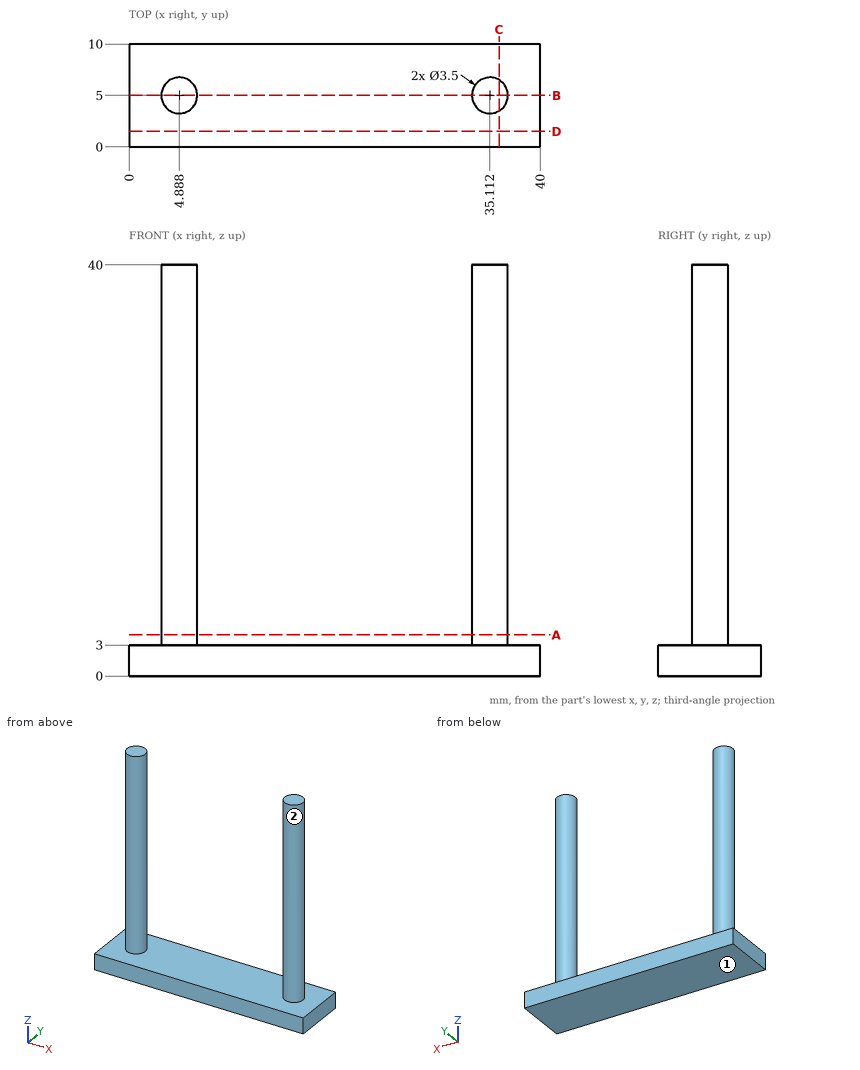
The drawing under review shows one solid part. Ordinate dimensions are in mm from its lowest x, y, z. Give positions to 0.01 mm unless a question says otherwise; leave off trailing zeros. Write each loop counter-clockwise with the first axis right and the second up, starting at its lowest first coordinate (ties: lowest second). Pieces come first, ordered by that corner, then holes.
1. Add section A-A, the plane z = 4. Write out the cut boundary in (x, y).
2. Add section C-C, the plane x = 36. Write out the cut boundary in (y, z).
3. Wall thickness on L1, parallel to Z at x = 15, y = 7.5; L2, parallel to Y at x = 35, z = 30; L3, parallel to X at y = 4.25, z = 23: over which ranges is each line inside the solid? List them lowest first.
4. For P1, Ø6, axis at y = 8.5, z = 35, coming from the +X side; P2, Ø12, axis at x = 17.5, z = 13, coming from the +Y side; P3, Ø5, axis at y = 7.5, z = 16.5, coming from the -X side, all flat-tipped, find the tip position at first contact; note any pin that passes through.
5. Draft analysis for pull direction X (two halves, no side actions). For the marked faces 1 and 2, state which applies: +X half, -X half, draft (parallel to the pull), parting line (faces both ways), or undercut.
6. Add section B-B, the plane y = 5. Write out the cut boundary in (x, z).
7. Add section D-D, the plane y = 1.5. Write out the cut boundary in (x, z).
Worked answers:
1. outline: circle Ø3.5 at (4.89, 5); circle Ø3.5 at (35.11, 5)
2. outline: (0, 0) - (10, 0) - (10, 3) - (6.51, 3) - (6.51, 40) - (3.49, 40) - (3.49, 3) - (0, 3) - close
3. L1: z = 0 to 3
3. L2: y = 3.25 to 6.75
3. L3: x = 3.31 to 6.47, 33.53 to 36.69
4. P1: stops at x = 36.79
4. P2: passes through
4. P3: stops at x = 3.14
5. face 1: draft
5. face 2: undercut
6. outline: (0, 0) - (40, 0) - (40, 3) - (36.86, 3) - (36.86, 40) - (33.36, 40) - (33.36, 3) - (6.64, 3) - (6.64, 40) - (3.14, 40) - (3.14, 3) - (0, 3) - close
7. outline: (0, 0) - (40, 0) - (40, 3) - (0, 3) - close
